```python
from build123d import *

# Parameters (mm, degrees)
F0_W     = 76.0293379426
F0_H     = 80.7674229145
F1_DEPTH = 42.164
F1_TAPER = -3
F2_R     = 13.0264691776
F3_DEPTH = 117.094
F4_R     = 5.5188922036


with BuildPart() as f1:
    # F0 (on Front) → F1 (new body)
    with BuildSketch(Plane.XZ):
        with Locations((-6.2791183591, 2.6857145131)):
            Rectangle(F0_W, F0_H)
    extrude(amount=F1_DEPTH, taper=F1_TAPER)

    # F2 (on face) → F3 (join)
    with BuildSketch(Plane.XZ.offset(42.164)):
        with Locations((-25.1841899008, -16.8737992644)):
            Circle(F2_R)
    extrude(amount=F3_DEPTH)

    # F4
    f4_edges = [f1.edges().sort_by_distance(p)[0] for p in [
        (-38.210659, -159.258, -16.873799),
    ]]
    fillet(f4_edges, radius=F4_R)


solid = f1.part
```
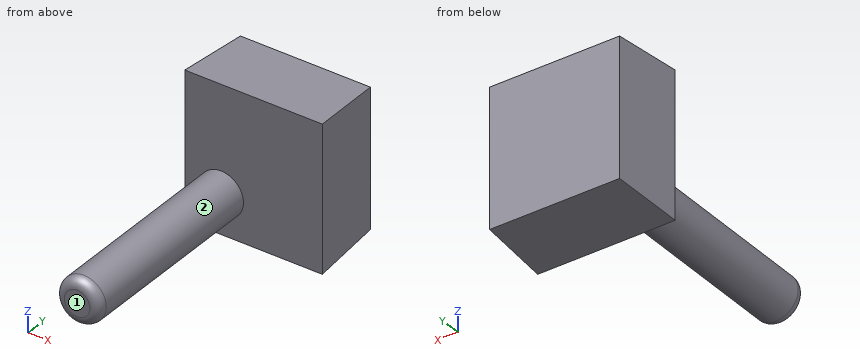
Could you check a few things on this model? Use its own coordinates, in mm. Face numbers are marked on the shaded views. A direction names the side the tool comes from. Coordinates: 2 decimals unless noted, no trailing zeros. Write each loop counter-clockwise with the first axis right and the second up, starting at its lowest first coordinate (ties: lowest second). Pieces come first, ordered by that corner, then holes. Notation, with made-up numbers: (88, 35) -> (145, 35) arc R20 ccw to (145, 49) -> close; hole circle Ø4 at (62.5, -40). An arc over 180 degrees is marked (long way). Write item = value, one per line. Start each with the question number.
(1) Which directions (+Z, -Z, +X, -X, +Y, -Y) give clear straight access to the entire face, cutting with the end or side of a thin tool? Please do the marked faces 1 and 2.
(2) I want a section at A-A (y = -133). Please give me the cut outline in (x, z), plus the area to 3 significant figures.
(3) I need wall thicknesses on line 1 (Y direction, x = 22.5, z = 37.5); line 2 (X direction, y = -61, z = -17); line 3 (X direction, y = -28, z = 0.5). Which ranges of each line are inside material? Lowest first, please. Write a range as [from, to].
(4) Will these pins go through, and if not, where does the flat tip stop? pin 1 (24 mm diameter, centred on x = -18, z = 16.5, fed in from -Y); pin 2 (8 mm diameter, centred on x = -33, y = -103, fed in from -Z); pin 3 (1.5 mm diameter, centred on y = -141, z = -10, fed in from -X).
Result set:
q1.face_1 = +Z, -Z, +X, -X, -Y
q1.face_2 = -Y
q2.outline = circle Ø26.05 at (-25.18, -16.87)
q2.area = 533 mm2
q3.line_1 = [-42.16, 0]
q3.line_2 = [-38.21, -12.16]
q3.line_3 = [-45.76, 33.2]
q4.pin_1 = -42.16
q4.pin_2 = -29.33
q4.pin_3 = -36.68
